Part print with two shaded views. Sizes in mm from the minimum x, y, z corner. Coordinates: 2 decimals unless noted, no trailing zeros. Write each loop counter-clockwise with the first axis right and the second up, starting at its lowest first coordinate (ties: lowest second). Pieces come first, ordered by that corner, then holes. Notation, with made-up numbers: (19, 35.5) - (47, 35.5) arc R16 cw to (47, 46.5) - close; hole circle Ø2 at (36.25, 73.5). An arc over 180 degrees is marked (long way). One line per question, with ' | ' between items. Start each with the question number.
1. Band-saw the part on B-B, the plane z = 12.5. Write the cut outline in (x, y), then the cut area to 3 significant figures.
2. Band-saw the part on A-A, the plane x = 12.5. Write the cut outline in (y, z).
3. Flat gauge pins, fed straight in: P1, Ø4, axis at y = 7.5, z = 10.5, coming from the +X side; P2, Ø5, axis at y = 6.5, z = 22, coming from the -X side; P3, Ø1.5, axis at x = 10.5, y = 9, coming from the +Z side; P4, Ø12.5, axis at x = 16.5, z = 17, coming from the -Y side. Where does each tip first touch, or does it go through?
4. Probe line 1 (Z direction, x = 12.5, y = 6.25); line 2 (Y direction, x = 19.25, z = 22); line 3 (Z direction, x = 8.25, y = 2). List the from-to ranges inside material, lowest first.
5. Band-saw the part on C-C, the plane y = 3.5. Write the cut outline in (x, z).
6. Two-plate mould, pull along X, no slides. Class the marked faces 1, 2 and 3: +X half, -X half, draft (parallel to the pull), parting line (faces both ways), or undercut.
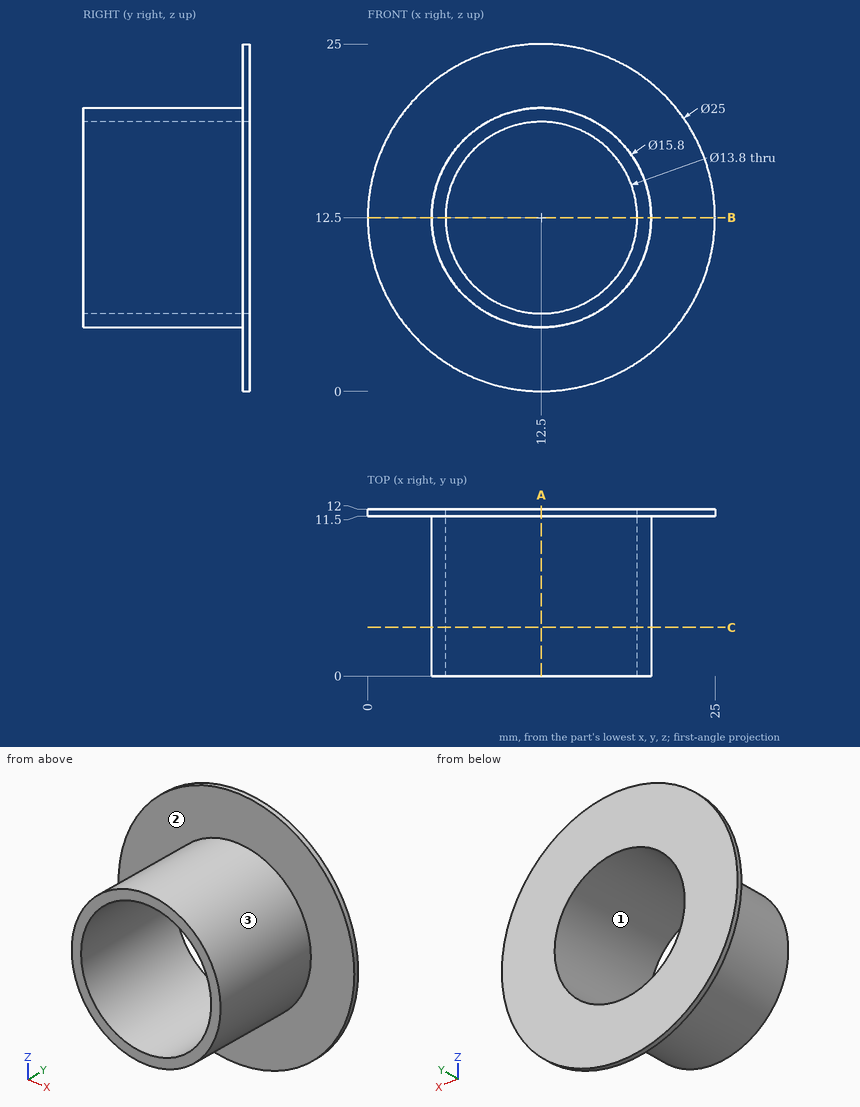
Filled in:
1) outline: (0, 11.5) - (4.6, 11.5) - (4.6, 0) - (5.6, 0) - (5.6, 12) - (0, 12) - close; (19.4, 0) - (20.4, 0) - (20.4, 11.5) - (25, 11.5) - (25, 12) - (19.4, 12) - close | area: 28.6 mm²
2) outline: (0, 4.6) - (11.5, 4.6) - (11.5, 0) - (12, 0) - (12, 5.6) - (0, 5.6) - close; (0, 19.4) - (12, 19.4) - (12, 25) - (11.5, 25) - (11.5, 20.4) - (0, 20.4) - close
3) P1: stops at x = 20.4 | P2: stops at x = 8.84 | P3: stops at z = 20.3 | P4: stops at y = 0
4) line 1: z = 4.6 to 5.6, 19.4 to 20.4 | line 2: y = 11.5 to 12 | line 3: z = 5.84 to 7.06, 17.94 to 19.16
5) outline: circle Ø15.8 at (12.5, 12.5); hole circle Ø13.8 at (12.5, 12.5)
6) face 1: undercut | face 2: draft | face 3: parting line
